For this review, take the finished solid that the model builds, in its own axes (mm). A direction names the side the tool comes from. Round coordinates to 2 decimals unless told otherwise and drop trailing zeros. Write each loop counter-clockwise with the first axis right and the second up, starting at its lowest first coordinate (ties: lowest second). Pieces come first, ordered by that corner, then holes. Notation, with made-up numbers: (-13.75, 34) -> (-1.75, 34) arc R23 cw to (-1.75, 62) -> close; hole circle Ø5 at (4, -33.75). An arc over 180 degrees is marked (long way). Write item = value, one per line. Start each with the question number.
Autodesk Inventor part; units mm, degrees
ref_plane "YZ Plane" through (0, 0, 0) normal (1, 0, 0) x (0, 1, 0)
ref_plane "XZ Plane" through (0, 0, 0) normal (0, 1, 0) x (-1, 0, 0)
ref_plane "XY Plane" through (0, 0, 0) normal (0, 0, 1) x (1, 0, 0)
sketch "草图1" plane through (0, 0, 0) normal (0, 1, 0) x (-1, 0, 0)
  circle A0 centre (0, 0) radius 650
  dimension "d0" = 1300
extrude "拉伸1" add sketch "草图1" along normal blind 30
sketch "草图2" plane through (0, 0, 0) normal (1, 0, 0) x (0, 1, 0)
  line L0 (0, 570) -> (-30, 570)
  line L1 (-30, 570) -> (-30, 600)
  line L2 (-30, 600) -> (0, 600)
  line L3 (0, 600) -> (0, 570)
  line L4 (0, -650) -> (0, 650)
  point P0 (0, 0)
  dimension "d3" = 30
  dimension "d4" = 30
  dimension "d7" = 50
sketch "草图3" plane through (0, 0, 0) normal (0, -1, 0) x (1, 0, 0)
  circle A0 centre (0, 0) radius 600
  dimension "d8" = 1200
sweep "扫掠1" add profiles "草图2" path "草图3"
sketch "草图4" plane through (0, 0, 0) normal (0, 0, 1) x (1, 0, 0)
  line L0 (-600, -30) -> (600, -30)
  line L1 (-570, -30) -> (570, -30)
  line L2 (600, -30) -> (570, -30)
  line L3 (575, -60) -> (595, -60)
  line L4 (570, -55) -> (570, -50)
  line L5 (570, -30) -> (570, -40)
  arc A0 (570, -50) -> (570, -40) centre (570, -45) ccw
  arc A1 (600, -40) -> (600, -50) centre (600, -45) ccw
  line L6 (600, -55) -> (600, -50)
  line L7 (600, -40) -> (600, -30)
  line L8 (575, -60) -> (570, -55)
  line L9 (595, -60) -> (600, -55)
  point P0 (0, 0)
  point P1 (570, -60)
  point P2 (600, -60)
  dimension "d12" = 10
  dimension "d13" = 10
  dimension "d14" = 5
  dimension "d15" = 5
  dimension "d16" = 5
  dimension "d17" = 5
  dimension "d18" = 5
sketch3d "三维草图1"
  arc A0 (570, -30, 0) -> (0, -30, 570) centre (0, -30, 0) ccw
  arc A1 (0, -30, 570) -> (-570, -30, 0) centre (0, -30, 0) ccw
  arc A2 (-570, -30, 0) -> (0, -30, -570) centre (0, -30, 0) ccw
  arc A3 (0, -30, -570) -> (570, -30, 0) centre (0, -30, 0) ccw
sweep "扫掠2" add profiles "草图4" path "三维草图1"
sketch "草图6" plane through (0, 30, 0) normal (0, 1, 0) x (1, 0, 0)
  circle A0 centre (0, 0) radius 650
  circle A1 centre (0, 0) radius 650
  circle A2 centre (0, 0) radius 600
extrude "拉伸3" add sketch "草图6" along normal blind 100
sketch "草图7" plane through (0, 30, 0) normal (0, 1, 0) x (1, 0, 0)
  circle A0 centre (0, 0) radius 100
  dimension "d35" = 200
extrude "拉伸4" add sketch "草图7" along normal blind 1000
sketch "草图8" plane through (0, 0, 0) normal (0, -1, 0) x (1, 0, 0)
  circle A0 centre (0, 0) radius 15
  dimension "d38" = 30
sketch "草图9" plane through (0, 0, 0) normal (0, -1, 0) x (1, 0, 0)
  point P0 (0, 0)
extrude "拉伸5" cut sketch "草图8" against normal blind 50
scale "缩放比例1" factors (0.4, 0.4, 0.4) then translate (0, 0, 0) bodies 1
sketch "草图10" plane through (0, 12, 0) normal (0, 1, 0) x (1, 0, 0)
  circle A0 centre (0, 0) radius 6
  line L0 (0, 0) -> (240, 0)
  circle A1 centre (0, 0) radius 240
  line L1 (0, 0) -> (74.1641, 228.2536)
  line L2 (0, 0) -> (-194.1641, 141.0685)
  line L3 (0, 0) -> (-194.1641, -141.0685)
  line L4 (0, 0) -> (74.1641, -228.2536)
  circle A2 centre (0, 0) radius 50
  line L5 (0, -5) -> (240, -5)
  line L6 (0, 5) -> (240, 5)
  point P0 (239.9479, 5)
  point P1 (49.7494, 5)
  point P2 (49.7494, -5)
  point P3 (239.9479, -5)
  dimension "d46" = 360
  dimension "d48" = 100
  dimension "d49" = 5
  dimension "d50" = 5
extrude "拉伸6" add sketch "草图10" along normal blind 30 contours A2 L6 A1 L0 | L0 A1 L5 A2
pattern_circular "环形阵列2" count 5 over 360 about axis through (0, 12, 0) along (0, 1, 0) of "拉伸6"
extrude "拉伸7" add sketch "草图10" along normal blind 40 contours L0 A2 L5 A0 | A0 L6 A2 L0 | A0 L1 A2 L6 | L5 A2 L4 A0 | A0 L2 A2 L1 | L4 A2 L3 A0 | A0 L3 A2 L2
scale "缩放比例2" factors (1.25, 1.25, 1.25) then translate (0, 0, 0) bodies 1
properties part number "上导轨"
1. Draft analysis for pull direction Z (two halves, no side actions). For faces 4 (the cylindrical face through (138.432, -9.86, 266.152)), 5 (the flat face through (61.38, 33.49, -168.68)), 6 (the flat face through (-95, 0, -287)), state which applies: +Z half, -Z half, draft (parallel to the pull), parting line (faces both ways), or undercut.
2. Machinability: for faces 1 (the cylindrical face through (266.152, -26.232, -138.432)), 2 (the flat face through (282, -30, 62)), 3 (the flat face through (164, 15, -112)), which of the approach directions +Z, -Z, +X, -X, +Y, -Y give a long, thin tool a straight path to every point of the face, cutting with its end or side? Answer none if there is none.
3. Clearance check with flat-ended pins moving along their axes: pin 1 Ø14 at (x, z) = (231.5, 1.5) entering from +Y; pin 2 Ø6 at (x, z) = (-31, 165) entering from +Y. State where each tip first meets the part, or that it passes through.
4. Wall thickness on L1, parallel to Z at x = 0, y = 21.5; L2, parallel to Z at x = 0, y = -27: over which ranges is each line inside the solid? List them lowest first. Write a range as from..to.
5. Consider section A-A, the plane y = 286. Give the boundary of the cut face in (x, z), then the cut area to 3 significant figures.
Outcome:
q1.face_4 = parting line
q1.face_5 = undercut
q1.face_6 = draft
q2.face_1 = -Y
q2.face_2 = +Z, -Z, +X, -X, -Y
q2.face_3 = +Y
q3.pin_1 = 52.5
q3.pin_2 = 15
q4.L1 = -325..-300, -62.5..-7.5, 7.5..62.5, 300..325
q4.L2 = -300..-285, 285..300
q5.outline = circle Ø100 at (0, 0)
q5.area = 7,850 mm2
